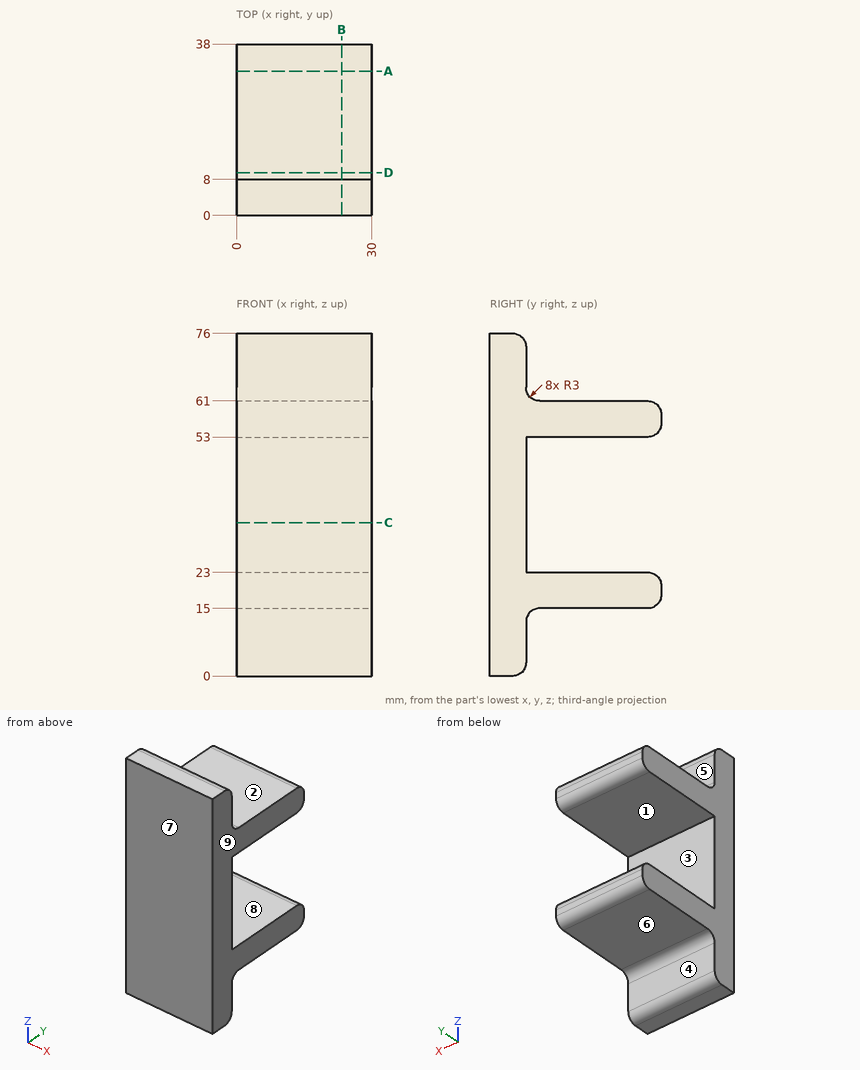
For this review, use the dimensioned drawing (mm, ordinates from the lowest corner) and the shaded views. A direction names the side the tool comes from. Round coordinates to 2 decimals unless told otherwise and drop trailing zeros. Write each loop counter-clockwise with the first axis right and the second up, starting at its lowest first coordinate (ties: lowest second). Pieces come first, ordered by that corner, then holes. Notation, with made-up numbers: (7.5, 42.5) -> (33.5, 42.5) arc R27 ccw to (33.5, 65.5) -> close; hole circle Ø7 at (-5.75, -24). An arc over 180 degrees is marked (long way). One line per item, written item: value. Start each with the question number.
Q1. Add section B-B (x = 23.25). Give the boundary of the cut face in (y, z), then the cut area to 3 significant figures.
Q2. To check wall thickness, follow probe 1 along Z at (x, y) = (15.75, 20.5); probe 2 along Y at (x, z) = (24.5, 34); probe 3 along Z at (x, y) = (7, 6). State the ranges of each line that lie inside material, in increasing order.
Q3. Add section D-D (y = 9.5). Give the boundary of the cut face in (x, z), then the cut area to 3 significant figures.
Q4. Insertion check: P1, Ø2, axis at x = 22, z = 37, coming from the +Y side; P2, Ø7, axis at x = 11, y = 18, coming from the +Z side; P3, Ø3, axis at y = 16.5, z = 16, coming from the -X side; P4, Ø12, axis at x = 12, y = 26, coming from the -Z side. Each pin has a flat end and moves straight along its axis. Give the tip position at first contact, or say it passes through.
Q5. The part is to be moulded in two halves that separate along Z. For the marked faces 1, 2, 3 and 4, say which applies: pulls with the +Z half, pulls with the -Z half, needs draft (parallel to the pull), parting line crosses it, or undercut.
Q6. Tool access review of the marked faces 5, 6, 7, 8 and 9: name each direction out of +Z, -Z, +X, -X, +Y, -Y from which nothing blocks a thin tool from reaching the whole face with its end or side.
Q7. Add section A-A (y = 32). Give the boundary of the cut face in (x, z), then the cut area to 3 significant figures.
Q8. Add section C-C (z = 34). Give the boundary of the cut face in (x, y), then the cut area to 3 significant figures.
Response:
1. outline: (0, 0) -> (5, 0) arc R3 ccw to (8, 3) -> (8, 12) arc R3 cw to (11, 15) -> (35, 15) arc R3 ccw to (38, 18) -> (38, 20) arc R3 ccw to (35, 23) -> (8, 23) -> (8, 53) -> (35, 53) arc R3 ccw to (38, 56) -> (38, 58) arc R3 ccw to (35, 61) -> (11, 61) arc R3 cw to (8, 64) -> (8, 73) arc R3 ccw to (5, 76) -> (0, 76) -> close
1. area: 1,080 mm^2
2. probe 1: z = 15 to 23, 53 to 61
2. probe 2: y = 0 to 8
2. probe 3: z = 0.17 to 75.83
3. outline: (0, 14.6) -> (30, 14.6) -> (30, 23) -> (0, 23) -> close; (0, 53) -> (30, 53) -> (30, 61.4) -> (0, 61.4) -> close
3. area: 504 mm^2
4. P1: stops at y = 8
4. P2: stops at z = 61
4. P3: stops at x = 0
4. P4: stops at z = 15
5. face 1: undercut
5. face 2: pulls with the +Z half
5. face 3: undercut
5. face 4: needs draft
6. face 5: +Z, +X, -X, +Y
6. face 6: -Z, +X, -X, +Y
6. face 7: +Z, -Z, +X, -X, -Y
6. face 8: +X, -X, +Y
6. face 9: +Z, -Z, +X, +Y, -Y
7. outline: (0, 15) -> (30, 15) -> (30, 23) -> (0, 23) -> close; (0, 53) -> (30, 53) -> (30, 61) -> (0, 61) -> close
7. area: 480 mm^2
8. outline: (0, 0) -> (30, 0) -> (30, 8) -> (0, 8) -> close
8. area: 240 mm^2
